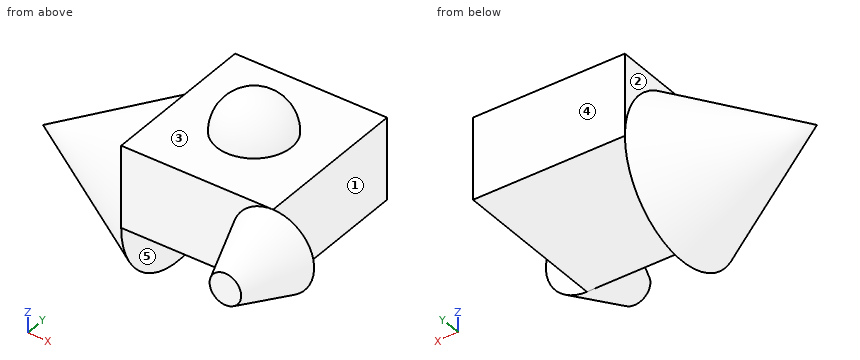
from build123d import *

# Parameters (mm, degrees)
F0_W     = 46.27084
F0_H     = 48.0736
F1_DEPTH = 12.5


with BuildPart() as f1:
    # F0 (on Top) → F1 (new body, symmetric)
    with BuildSketch(Plane.XY):
        Rectangle(F0_W, F0_H)
    extrude(amount=F1_DEPTH, both=True)

    # F2 (on face) → F3 (revolve)
    with BuildSketch(Plane.XY.offset(12.5)):
        with BuildLine():
            Line((0, 0), (-11.412725, 0))
            ThreePointArc((-11.412725, 0), (0, -11.412725), (11.412725, 0))
            Line((11.412725, 0), (0, 0))
        make_face()
    revolve(axis=Axis((0, 0, 12.5), (-1, 0, 0)))

    # F4 (on face) → F5 (revolve)
    with BuildSketch(Plane(origin=(0, 0, -12.5), x_dir=(1, 0, 0), z_dir=(0, 0, -1))):
        Polygon((-64.298436, 0), (-23.13542, -24.0368), (-23.13542, 0), align=None)
    revolve(axis=Axis((-43.716928, 0, -12.5), (1, 0, 0)))

    # F6 (on face) → F7 (revolve)
    with BuildSketch(Plane.YZ.offset(23.13542)):
        Polygon((-44.167623, -4.807361), (-24.0368, -12.5), (-24.0368, 0), (-44.167623, 0), align=None)
    revolve(axis=Axis((23.13542, -34.102212, 0), (0, 1, 0)))


solid = f1.part
Here's how the part is built. I have some questions about the finished solid (model axes, mm). Face numbers are marked on the shaded views. A direction names the side the tool comes from. Coordinates: 2 decimals unless noted, no trailing zeros. Order: outer loops, then holes, each group sorted by start corner. A loop starts at its lowest first (then second) coordinate and runs counter-clockwise, first axis right, second up.
Item 1: If we section it at A-A on x = -0.5: List the corners of the cut face in (y, z) for me.
Result sheet:
outline: (-24.04, -12.5) - (24.04, -12.5) - (24.04, 12.5) - (11.4, 12.5) arc R11.4 ccw to (-11.4, 12.5) - (-24.04, 12.5) - close
Item 2: If we section it at C-C on x = -28: List the corners of the cut face in (y, z) for me.
Result sheet:
outline: circle Ø42.39 at (0, -12.5)
Item 3: If we section it at B-B on y = -31.5: List the corners of the cut face in (x, z) for me, plus the area to 3 significant figures.
Result sheet:
outline: circle Ø19.3 at (23.14, 0)
area: 292 mm2
Item 4: I need wall thicknesses on line 1 (Y direction, x = 8, z = 5); line 2 (Z direction, x = -27, y = 9.5); line 3 (X direction, y = 13.5, z = 8). Which ranges of each line are inside material? Lowest first, please.
Result sheet:
line 1: y = -24.04 to 24.04
line 2: z = -32.1 to 7.1
line 3: x = -23.14 to 23.14
Item 5: For P1, Ø14, axis at x = 6.5, y = -10.5, coming from the -Z side; P2, Ø10, axis at x = -48.5, z = 0, coming from the -Y side; P3, Ø1.5, axis at x = -28.5, z = -27, coming from the -Y side, each with a flat end and sliding along its axis, tell me the tip position at first contact or that it passes through.
Result sheet:
P1: stops at z = -12.5
P2: stops at y = -6.95
P3: stops at y = -15.97
Item 6: For the marked faces 1, 2, 3, 4 and 5, which set-ups out of +Z, -Z, +X, -X, +Y, -Y let a thin tool reach every point of the face, with its end or its side?
Result sheet:
face 1: +Z, -Z, +X, +Y
face 2: +Z, -X
face 3: +Z
face 4: +Z, -Z, +X, -X, +Y
face 5: -Z, +X, +Y, -Y
